Geometry check sheet. Reference: the model listing, model coordinates, mm. A direction names the side the tool comes from. Give positions to 0.01 mm unless a question says otherwise; leave off trailing zeros. Write each loop counter-clockwise with the first axis right and the second up, starting at its lowest first coordinate (ties: lowest second). Pieces come first, ordered by that corner, then holes. Notation, with made-up numbers: M 33,83.5 L 73,83.5 A8 cw 73,94.5 Z; hole C 25,75.25 d8. An arc over 180 degrees is marked long. One line per item, written item: value. Start each with the question number.
1. Gauge pin test, flat ends, axial feed: pin 1 (2 mm diameter, centred on x = -8, y = -7.5, fed in from +Z); pin 2 (0.9 mm diameter, centred on x = 6, y = -4, fed in from -Z); pin 3 (1.1 mm diameter, centred on x = -6, z = 7, fed in from -Y). Record the tip position at first contact, or that the pin passes through.
2. Cross-section at A-A on z = 4.5. Record the cut outline in (x, y) (3 decimals).
3. Scan lines: line 1 (Z direction, x = 8, y = -3.5); line 2 (Z direction, x = 4.5, y = -2.5); line 3 (X direction, y = -7, z = 2). Record each from-to range of solid material in increasing order.
4. Release check for a two-part mould opening along Y. For faces 1 (the face through (-2.524, -7.597, 4.208)), 2 (the face through (4.314, -2.472, 3.715)), 3 (the face through (6.307, -4.305, 6.989)), 4 (the face through (2.564, -7.528, 4.208)) record: pulls with the +Y half, pulls with the -Y half, needs draft (parallel to the pull), parting line crosses it, or undercut.
5. Cross-section at C-C on x = 0. Record the cut outline in (y, z).
6. Cross-section at B-B on y = -4. Record the cut outline in (x, z).
7. Tool access check on faces 5 (the face through (7, -5, -1)), 6 (the face through (-4.314, -7.528, 3.715)), 7 (the face through (-5, -5.125, 4)), 8 (the face through (-5.8, -3.75, 6.8)). Record the directions out of +Z, -Z, +X, -X, +Y, -Y that give a thin tool (end or side, any length) a straight path to the whole face; none if there is none.
8. Cross-section at D-D on y = -5.5. Record the cut outline in (x, z).
from build123d import *

# Parameters (mm, degrees)
F1_DEPTH    = 10
F3_DEPTH    = 6
F6_DEPTH    = 1
F7_DEPTH    = 1
F8_T1_DEPTH = 11.1602540378
F9_R        = 1
F10_W       = 3.6315133076
F10_H       = 0.25
F11_DEPTH   = 6
F12_W       = 3.6315133076
F12_H       = 0.25
F13_DEPTH   = 6


# Not quite as in the source:
# - a fillet or chamfer that OpenCascade refuses, or shapes differently, is made with other operations: its cross-section is extruded or revolved along the edge and cut away or added


with BuildPart() as f1:
    # F0 (on Front) → F1 (new body)
    with BuildSketch(Plane.XZ):
        Polygon((7, -1.25), (10.5, -1.25), (10.5, 1.25), (-10.5, 1.25), (-10.5, -1.25), (-7, -1.25), (-7, -0.3903658071), (-9, -0.3903658071), (-9, 0.2096341929), (9, 0.2096341929), (9, -0.3903658071), (7, -0.3903658071), align=None)
    extrude(amount=F1_DEPTH)

    # F2 (on face) → F3 (join)
    with BuildSketch(Plane.XY.offset(1.25)):
        Polygon((-1.137, -10), (-4.0235, -5), (-5.7735, -5), (-2.887, -10), align=None)
        Polygon((-4.0235, -5), (-1.137, 0), (-2.887, 0), (-5.7735, -5), align=None)
        Polygon((2.887, 0), (1.137, 0), (4.0235, -5), (5.7735, -5), align=None)
        Polygon((5.7735, -5), (4.0235, -5), (1.137, -10), (2.887, -10), align=None)
    extrude(amount=F3_DEPTH)

    # F4 (on face) → F6 (join)
    with BuildSketch(Plane.XY.offset(7.25)):
        Polygon((-5.7735, -5), (-5.051875, -3.75), (-7.051875, -3.75), (-7.051875, -6.25), (-5.051875, -6.25), align=None)
    extrude(amount=-F6_DEPTH)

    # F5 (on face) → F7 (join)
    with BuildSketch(Plane.XY.offset(7.25)):
        Polygon((7.051875, -3.75), (5.051875, -3.75), (5.7735, -5), (5.051875, -6.25), (7.051875, -6.25), align=None)
    extrude(amount=-F7_DEPTH)

    # F8: fillet of radius 2 on 2 edges, made by hand

    # F8_s2 → F8_t1 (cut)
    with BuildSketch(Plane.XZ.offset(-0.5801270189)):
        with BuildLine():
            ThreePointArc((-5.3198241924, 7.25), (-6.3198241924, 6.9820508076), (-7.051875, 6.25))
            Line((-7.051875, 6.25), (-7.051875, 7.25))
            Line((-7.051875, 7.25), (-5.3198241924, 7.25))
        make_face()
        with BuildLine():
            ThreePointArc((5.3198241924, 7.25), (6.3198241924, 6.9820508076), (7.051875, 6.25))
            Line((7.051875, 6.25), (7.051875, 7.25))
            Line((7.051875, 7.25), (5.3198241924, 7.25))
        make_face()
    extrude(amount=F8_T1_DEPTH, mode=Mode.SUBTRACT)

    # F9
    f9_edges = [f1.edges().sort_by_distance(p)[0] for p in [
        (-3.969438, -8.125, 7.25),
        (-3.969438, -1.875, 7.25),
        (3.969437, -8.125, 7.25),
        (3.969437, -1.875, 7.25),
    ]]
    fillet(f9_edges, radius=F9_R)

    # F10 (on face) → F11 (cut)
    with BuildSketch(Plane.XY.offset(7.25)):
        Polygon((-4.0235, -5), (-3.9513375, -4.875), (-5.3198241924, -4.875), (-5.3198241924, -5.125), (-3.9513375, -5.125), align=None)
        with Locations((-7.1355808462, -5)):
            Rectangle(F10_W, F10_H)
    extrude(amount=-F11_DEPTH, mode=Mode.SUBTRACT)

    # F12 (on face) → F13 (cut)
    with BuildSketch(Plane.XY.offset(7.25)):
        with Locations((7.1355808462, -5)):
            Rectangle(F12_W, F12_H)
        Polygon((5.3198241924, -4.875), (3.9513375, -4.875), (4.0235, -5), (3.9513375, -5.125), (5.3198241924, -5.125), align=None)
    extrude(amount=-F13_DEPTH, mode=Mode.SUBTRACT)


solid = f1.part
Report:
1. pin 1: stops at z = 1.25
1. pin 2: stops at z = 0.21
1. pin 3: stops at y = -6.25
2. outline: M -5.701,-5.125 L -2.887,-10 L -1.137,-10 L -3.951,-5.125 Z; M -5.701,-4.875 L -3.951,-4.875 L -1.137,0 L -2.887,0 Z; M 1.137,-10 L 2.887,-10 L 5.701,-5.125 L 3.951,-5.125 Z; M 1.137,0 L 3.951,-4.875 L 5.701,-4.875 L 2.887,0 Z
3. line 1: z = -1.25 to -0.39, 0.21 to 1.25
3. line 2: z = 0.21 to 1.25
3. line 3: x = -4.62 to -2.87, 2.87 to 4.62
4. face 1: undercut
4. face 2: pulls with the +Y half
4. face 3: needs draft
4. face 4: undercut
5. outline: M -10,0.21 L 0,0.21 L 0,1.25 L -10,1.25 Z
6. outline: M -10.5,-1.25 L -7,-1.25 L -7,-0.39 L -9,-0.39 L -9,0.21 L 9,0.21 L 9,-0.39 L 7,-0.39 L 7,-1.25 L 10.5,-1.25 L 10.5,1.25 L 5.2,1.25 L 5.2,6.25 L 7.05,6.25 A2 ccw 5.32,7.25 L 3.45,7.25 L 3.45,1.25 L -3.45,1.25 L -3.45,7.25 L -5.32,7.25 A2 ccw -7.05,6.25 L -5.2,6.25 L -5.2,1.25 L -10.5,1.25 Z
7. face 5: -Z, +Y, -Y
7. face 6: -X, -Y
7. face 7: +Z, +X, -X
7. face 8: +Z, -X, +Y
8. outline: M -10.5,-1.25 L -7,-1.25 L -7,-0.39 L -9,-0.39 L -9,0.21 L 9,0.21 L 9,-0.39 L 7,-0.39 L 7,-1.25 L 10.5,-1.25 L 10.5,1.25 L 5.48,1.25 L 5.48,6.25 L 7.05,6.25 A2 ccw 5.32,7.25 L 3.73,7.25 L 3.73,1.25 L -3.73,1.25 L -3.73,7.25 L -5.32,7.25 A2 ccw -7.05,6.25 L -5.48,6.25 L -5.48,1.25 L -10.5,1.25 Z
